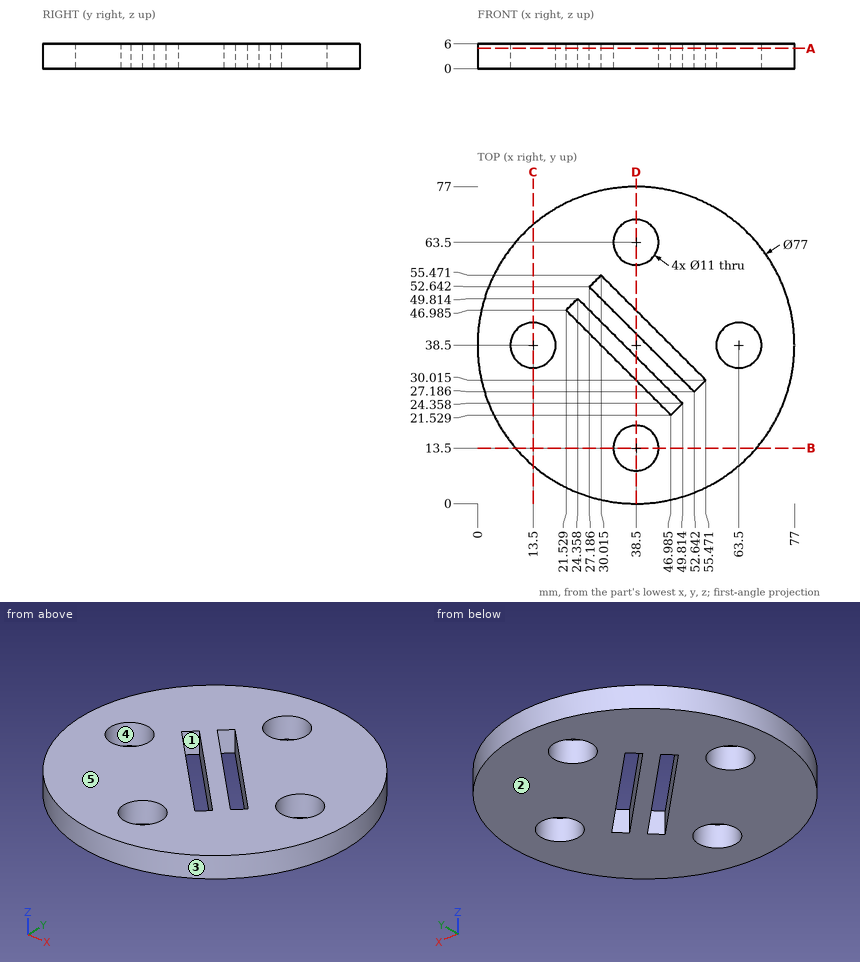
Verification items for this drawing (mm, ordinates from the low corner). A direction names the side the tool comes from. Coordinates: 2 decimals unless noted, no trailing zeros. Write each loop counter-clockwise with the first axis right and the second up, starting at its lowest first coordinate (ties: lowest second). Pieces come first, ordered by that corner, then holes. Notation, with made-up numbers: M -13,-9.75 L 41,-9.75 A6 cw 41,-4.75 Z; hole C 12.25,32 d3. An arc over 180 degrees is marked long. Answer as a JSON object with one key per item and string values. Group by question number.
(1) Tool access check on the marked faces 1 and 2. Record the directions out of +Z, -Z, +X, -X, +Y, -Y that give a thin tool (end or side, any length) a straight path to the whole face; none if there is none.
(2) Gauge pin test, flat end, axial feed: pin 1 (3 mm diameter, centred on y = 21.5, z = 3, fed in from +X). Record the tip position at first contact, or that the pin passes through.
(3) Cross-section at D-D, the plane x = 38.5. Record the cut outline in (y, z) (1 decimal), and give its area (3 significant figures).
(4) Cross-section at B-B, the plane y = 13.5. Record the cut outline in (x, z).
(5) Release check for a two-part mould opening along Y. For the marked faces 3, 4 and 5 record: +Y half, -Y half, draft (parallel to the pull), parting line (faces both ways), or undercut.
(6) Cross-section at A-A, the plane z = 4.95. Record the cut outline in (x, y) (1 decimal).
(7) Material ranges on line 1 (Y direction, x = 38.5, z = 1.7) (1 decimal); line 2 (X direction, y = 32.5, z = 1.1) (1 decimal); line 3 (X direction, y = 47.5, z = 2.85) (1 decimal), recorded low to high.
Reply:
{
 "1": {"face 1": "+Z, -Z", "face 2": "-Z, +X, -X, +Y, -Y"},
 "2": {"pin 1": "x = 73.74"},
 "3": {"outline": "M 0,0 L 8,0 L 8,6 L 0,6 Z; M 19,0 L 30,0 L 30,6 L 19,6 Z; M 35.7,0 L 41.3,0 L 41.3,6 L 35.7,6 Z; M 47,0 L 58,0 L 58,6 L 47,6 Z; M 69,0 L 77,0 L 77,6 L 69,6 Z", "area": "262 mm²"},
 "4": {"outline": "M 9.22,0 L 33,0 L 33,6 L 9.22,6 Z; M 44,0 L 67.78,0 L 67.78,6 L 44,6 Z"},
 "5": {"face 3": "parting line", "face 4": "undercut", "face 5": "draft"},
 "6": {"outline": "C 38.5,38.5 d77; hole C 13.5,38.5 d11; hole M 21.5,47 L 47,21.5 L 49.8,24.4 L 24.4,49.8 Z; hole M 27.2,52.6 L 52.6,27.2 L 55.5,30 L 30,55.5 Z; hole C 38.5,13.5 d11; hole C 38.5,63.5 d11; hole C 63.5,38.5 d11"},
 "7": {"line 1": "0 to 8, 19 to 30, 35.7 to 41.3, 47 to 58, 69 to 77", "line 2": "0.5 to 36, 41.7 to 47.3, 53 to 76.5", "line 3": "1.1 to 22, 26.7 to 32.3, 38 to 75.9"}
}
